Can you work these out from the model? Positions are in its coordinate system, mm. A direction names the side the tool comes from. Coordinates: 2 decimals unless noted, no trailing zeros. Write each loop counter-clockwise with the first axis right and the second up, starting at its lowest first coordinate (ties: lowest second). Pieces come first, ordered by that corner, then holes. Notation, with made-up numbers: (82, 63) - (107, 63) arc R22 cw to (107, 92) - close; hole circle Ø5 at (8, -30.5). An arc over 180 degrees is marked (long way). Use one line per item in the form item = value. Start each with the question number.
(1) If I drill on probe 1 along Y at (x, z) = (1, 94); probe 2 along Z at (x, y) = (1.5, 144); probe 3 along Z at (x, y) = (-9, 18), over which ranges is the centre line in solid material (lowest first)? Write a range as from..to.
(2) On a 3-axis mill with a long thin cutter (end or side, diameter ignored), from which of +Z, -Z, +X, -X, +Y, -Y can I reach the whole of each face in a straight line? I mean faces 1 (the face through (0, -3, 10)), 2 (the face through (12.5, 212, 85)), 3 (the face through (0, -226, 285)), 4 (the face through (-12.5, 212, 88)), 5 (the face through (-8, -3, 2)). Say none if no direction works.
(3) If we section it at B-B on y = 92: Please give me the cut outline in (x, z).
(4) Thinking about a two-plate mould opening in Y: for faces 6 (the face through (0, 217.5, 142)), 7 (the face through (8, -3, 2)), 8 (the face through (12.5, -212, 85)), which applies, pulls with the +Y half, pulls with the -Y half, needs draft (parallel to the pull), parting line crosses it, or undercut?
(5) For pin 1 Ø8 at (y, z) = (213.5, 133) entering from -X; pin 2 Ø1.6 at (x, y) = (-16, -214.5) entering from +Z; pin 3 Ø5 at (x, z) = (3.5, 185) entering from +Y, each with a flat end and sliding along its axis, tell me the tip position at first contact or that it passes through.
(6) If we section it at A-A on z = 226: Please give me the cut outline in (x, y).
```python
from build123d import *

# Parameters (mm, degrees)
PAD005_DEPTH = 12.5
PAD006_DEPTH = 10
PAD007_DEPTH = 10
SKETCH012_W  = 415
SKETCH012_H  = 16
PAD008_DEPTH = 8


with BuildPart() as part:
    # Sketch008 → Pad005 (new body, symmetric)
    with BuildSketch(Plane.YZ):
        Polygon((-235, 294), (235, 294), (235, 285), (207.5, 285), (207.5, 276), (-207.5, 276), (-207.5, 285), (-235, 285), align=None)
    extrude(amount=PAD005_DEPTH, both=True)

    # Sketch010 (on Face6 of Pad005) → Pad006 (join)
    with BuildSketch(Plane(origin=(0, -207.5, 0), x_dir=(0, 0, -1), z_dir=(0, -1, 0))):
        Polygon((-285, 18), (-285, -18), (-185, -18), (-179.5, -12.5), (6, -12.5), (6, 12.5), (-179.5, 12.5), (-185, 18), align=None)
    extrude(amount=PAD006_DEPTH)

    # Sketch011 (on Face8 of Pad006) → Pad007 (join)
    with BuildSketch(Plane.ZX.offset(207.5)):
        Polygon((-6, 12.5), (179.5, 12.5), (185, 18), (285, 18), (285, -18), (185, -18), (179.5, -12.5), (-6, -12.5), align=None)
    extrude(amount=PAD007_DEPTH)

    # Sketch012 → Pad008 (join, symmetric)
    with BuildSketch(Plane.YZ):
        with Locations((0, 2)):
            Rectangle(SKETCH012_W, SKETCH012_H)
    extrude(amount=PAD008_DEPTH, both=True)


solid = part.part
```
Reported:
q1.probe_1 = -217.5..-207.5, 207.5..217.5
q1.probe_2 = -6..10, 276..294
q1.probe_3 = 276..294
q2.face_1 = +X, -X
q2.face_2 = -Z, +X, +Y, -Y
q2.face_3 = -Z, +X, -X, -Y
q2.face_4 = -Z, -X, +Y, -Y
q2.face_5 = -Z, -X
q3.outline = (-12.5, 276) - (12.5, 276) - (12.5, 294) - (-12.5, 294) - close; (-8, -6) - (8, -6) - (8, 10) - (-8, 10) - close
q4.face_6 = pulls with the +Y half
q4.face_7 = undercut
q4.face_8 = needs draft
q5.pin_1 = -12.5
q5.pin_2 = 285
q5.pin_3 = 217.5
q6.outline = (-18, -217.5) - (18, -217.5) - (18, -207.5) - (-18, -207.5) - close; (-18, 207.5) - (18, 207.5) - (18, 217.5) - (-18, 217.5) - close
